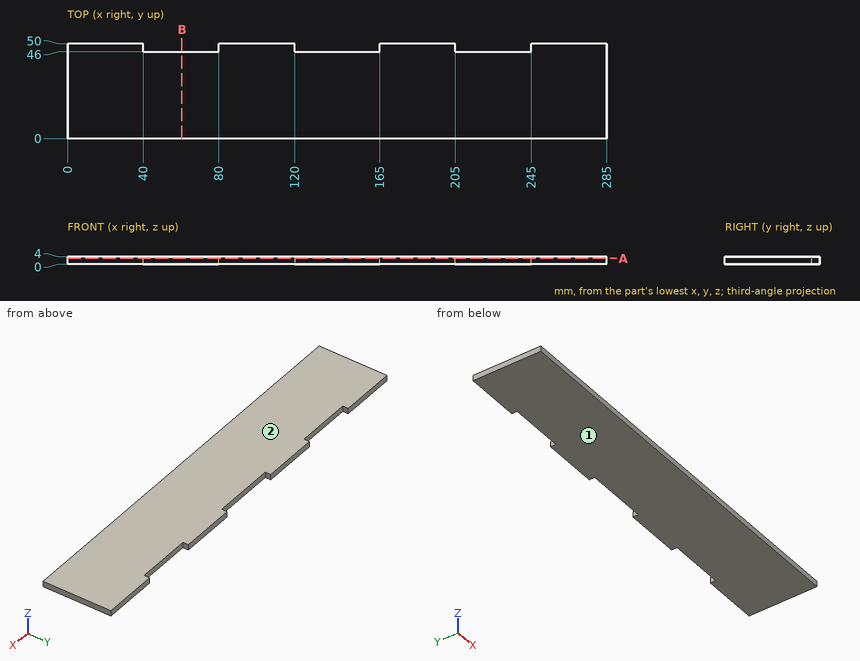
Verification items for this drawing (mm, ordinates from the low corner). Coordinates: 2 decimals unless noted, no trailing zeros. Loops run counter-clockwise (first coordinate to the right, second up) from the corner with the lowest first, then second, coordinate; pieces in that order, holes last. Notation, with made-up numbers: (-1, -1.5) - (41, -1.5) arc R13 cw to (41, 23.5) - close; hole circle Ø6 at (-17, 14.25). An arc over 180 degrees is marked (long way). One line per item, written item: value. Start each with the question number.
(1) Mould release check, pull along Z, two halves, no side actions. Record for the marked faces 1 and 2: released by +Z, released by -Z, zero draft, split by the parting line, or undercut.
(2) Cross-section at A-A on z = 3.1. Enter the section's corners in (x, y), plus the area to 4 significant figures.
(3) Cross-section at B-B on x = 60.5. Enter the section's corners in (y, z), plus the area to 3 significant figures.
(4) Material ranges on line 1 (X direction, y = 48.5, z = 1.1); line 2 (Y direction, x = 50, z = 2.15), recorded low to high. Write a range as [from, to].
(5) Depth check by flat-ended pin: P1, Ø2, axis at x = 232, z = 3, coming from the +Y side. Enter the tip coordinate at first touch or a pass-through.
Results below:
1. face 1: released by -Z
1. face 2: released by +Z
2. outline: (0, 0) - (285, 0) - (285, 50) - (245, 50) - (245, 46) - (205, 46) - (205, 50) - (165, 50) - (165, 46) - (120, 46) - (120, 50) - (80, 50) - (80, 46) - (40, 46) - (40, 50) - (0, 50) - close
2. area: 13,750 mm2
3. outline: (0, 0) - (46, 0) - (46, 4) - (0, 4) - close
3. area: 184 mm2
4. line 1: x = [0, 40], [80, 120], [165, 205], [245, 285]
4. line 2: y = [0, 46]
5. P1: stops at y = 46
